```python
from build123d import *

# Parameters (mm, degrees)
RESSALTO_EXTRUS_O1_DEPTH                            = 22.5
CHANFRO1_SIZE                                       = 9
CORTE_EXTRUS_O1_REACH                               = 24.5
ESBO_O3_W                                           = 1139.230904301
ESBO_O3_H                                           = 709.798033895
CORTE_EXTRUS_O5_DEPTH                               = 1.5
CORTE_EXTRUS_O6_REACH                               = 23
ESCAREADO_PARA_PARAFUSO_ALLEN_SEXTAVADO_D           = 4.5
ESCAREADO_PARA_PARAFUSO_ALLEN_SEXTAVADO_CSINK_D     = 8.96
ESCAREADO_PARA_PARAFUSO_ALLEN_SEXTAVADO_CSINK_ANGLE = 90
CORTE_EXTRUS_O7_DEPTH                               = 10


with BuildPart() as part:
    # Esboço1 → Ressalto-extrusão1 (new body, symmetric)
    with BuildSketch(Plane.XY):
        with BuildLine():
            Line((-62.301435521, 279.499553668), (62.301435521, 279.499553668))
            ThreePointArc((62.301435521, 279.499553668), (66.527618138, 278.562631538), (69.961879952, 275.927429764))
            Line((69.961879952, 275.927429764), (100.660444431, 239.342305259))
            ThreePointArc((100.660444431, 239.342305259), (102.396926208, 236.334630596), (103, 232.914429162))
            Line((103, 232.914429162), (103, 177.526516487))
            ThreePointArc((103, 177.526516487), (102.453136861, 174.425101506), (100.878507208, 171.697762944))
            Line((100.878507208, 171.697762944), (62.121492792, 125.508951777))
            ThreePointArc((62.121492792, 125.508951777), (60.546863139, 122.781613215), (60, 119.680198234))
            Line((60, 119.680198234), (60, 5.944191717))
            Line((60, 5.944191717), (52.319579452, -0.500446332))
            Line((52.319579452, -0.500446332), (-52.319579452, -0.500446332))
            Line((-52.319579452, -0.500446332), (-60, 5.944191717))
            Line((-60, 5.944191717), (-60, 119.680198234))
            ThreePointArc((-60, 119.680198234), (-60.546863139, 122.781613215), (-62.121492792, 125.508951777))
            Line((-62.121492792, 125.508951777), (-100.878507208, 171.697762944))
            ThreePointArc((-100.878507208, 171.697762944), (-102.453136861, 174.425101506), (-103, 177.526516487))
            Line((-103, 177.526516487), (-103, 232.914429162))
            ThreePointArc((-103, 232.914429162), (-102.396926208, 236.334630596), (-100.660444431, 239.342305259))
            Line((-100.660444431, 239.342305259), (-69.961879952, 275.927429764))
            ThreePointArc((-69.961879952, 275.927429764), (-66.527618138, 278.562631538), (-62.301435521, 279.499553668))
        make_face()
        Polygon((-52.721623425, 259.499553668), (52.721623425, 259.499553668), (83, 223.415189606), (83, 181.505464287), (35, 124.301291842), (35, 19.499553668), (-35, 19.499553668), (-35, 124.301291842), (-83, 181.505464287), (-83, 223.415189606), align=None, mode=Mode.SUBTRACT)
    extrude(amount=RESSALTO_EXTRUS_O1_DEPTH, both=True)

    # Chanfro1
    chanfro1_edges = [part.edges().sort_by_distance(p)[0] for p in [
        (0, -0.500446332, 22.5),
        (56.159789726, 2.721872692, 22.5),
        (60, 62.812194975, 22.5),
        (60.546863139, 122.781613215, 22.5),
        (81.5, 148.603357361, 22.5),
        (102.453136861, 174.425101506, 22.5),
        (103, 205.220472825, 22.5),
        (102.396926208, 236.334630596, 22.5),
        (85.311162192, 257.634867512, 22.5),
        (66.527618138, 278.562631538, 22.5),
        (0, 279.499553668, 22.5),
        (-66.527618138, 278.562631538, 22.5),
        (-85.311162192, 257.634867512, 22.5),
        (-102.396926208, 236.334630596, 22.5),
        (-103, 205.220472825, 22.5),
        (-102.453136861, 174.425101506, 22.5),
        (-81.5, 148.603357361, 22.5),
        (-60.546863139, 122.781613215, 22.5),
        (-60, 62.812194975, 22.5),
        (-56.159789726, 2.721872692, 22.5),
    ]]
    chamfer(chanfro1_edges, length=CHANFRO1_SIZE)

    # Esboço3 → Corte-extrusão1 (cut, up to next)
    with BuildSketch(Plane.XY, mode=Mode.PRIVATE) as corte_extrus_o1_sk1:
        with Locations((-153.157436203, 152.53565808)):
            Rectangle(ESBO_O3_W, ESBO_O3_H)
    corte_extrus_o1_tool1 = extrude(corte_extrus_o1_sk1.sketch, amount=-CORTE_EXTRUS_O1_REACH, mode=Mode.PRIVATE) & part.part
    add(corte_extrus_o1_tool1.solids().sort_by_distance((-153.157436, 152.535658, 0))[0], mode=Mode.SUBTRACT)

    # Esboço4 → Corte-extrusão5 (cut)
    with BuildSketch(Plane.XY.offset(22.5)):
        Polygon((62.301435521, 269.499553668), (-62.301435521, 269.499553668), (-93, 232.914429162), (-93, 177.865761944), (-50, 126.620357463), (-50, 10.607268298), (-48.679877109, 9.499553668), (48.679877109, 9.499553668), (50, 10.607268298), (50, 126.620357463), (93, 177.865761944), (93, 232.914429162), align=None)
        Polygon((35, 19.499553668), (-35, 19.499553668), (-35, 124.301291842), (-83, 181.505464287), (-83, 223.415189606), (-52.721623425, 259.499553668), (52.721623425, 259.499553668), (83, 223.415189606), (83, 181.505464287), (35, 124.301291842), align=None, mode=Mode.SUBTRACT)
    extrude(amount=-CORTE_EXTRUS_O5_DEPTH, mode=Mode.SUBTRACT)

    # Esboço5 → Corte-extrusão6 (cut, up to next)
    with BuildSketch(Plane.XY.offset(21), mode=Mode.PRIVATE) as corte_extrus_o6_sk1:
        Polygon((-93, 232.914429162), (-83, 223.415189606), (-83, 181.505464287), (-35, 124.301291842), (-35, 108.744053574), (-93, 177.865761944), align=None)
    corte_extrus_o6_tool1 = extrude(corte_extrus_o6_sk1.sketch, amount=-CORTE_EXTRUS_O6_REACH, mode=Mode.PRIVATE) & part.part
    add(corte_extrus_o6_tool1.solids().sort_by_distance((-88.943881, 227.171171, 21))[0], mode=Mode.SUBTRACT)
    # Esboço5 → Corte-extrusão6 (cut, up to next)
    with BuildSketch(Plane.XY.offset(21), mode=Mode.PRIVATE) as corte_extrus_o6_sk2:
        Polygon((-52.721623425, 259.499553668), (-62.301435521, 269.499553668), (62.301435521, 269.499553668), (52.721623425, 259.499553668), align=None)
    corte_extrus_o6_tool2 = extrude(corte_extrus_o6_sk2.sketch, amount=-CORTE_EXTRUS_O6_REACH, mode=Mode.PRIVATE) & part.part
    add(corte_extrus_o6_tool2.solids().sort_by_distance((0, 264.638364, 21))[0], mode=Mode.SUBTRACT)
    # Esboço5 → Corte-extrusão6 (cut, up to next)
    with BuildSketch(Plane.XY.offset(21), mode=Mode.PRIVATE) as corte_extrus_o6_sk3:
        Polygon((-50, 10.607268298), (-35, 19.499553668), (35, 19.499553668), (50, 10.607268298), (48.679877109, 9.499553668), (-48.679877109, 9.499553668), align=None)
    corte_extrus_o6_tool3 = extrude(corte_extrus_o6_sk3.sketch, amount=-CORTE_EXTRUS_O6_REACH, mode=Mode.PRIVATE) & part.part
    add(corte_extrus_o6_tool3.solids().sort_by_distance((0, 14.193497, 21))[0], mode=Mode.SUBTRACT)
    # Esboço5 → Corte-extrusão6 (cut, up to next)
    with BuildSketch(Plane.XY.offset(21), mode=Mode.PRIVATE) as corte_extrus_o6_sk4:
        Polygon((35, 108.744053574), (93, 177.865761944), (93, 232.914429162), (83, 223.415189606), (83, 181.505464287), (35, 124.301291842), align=None)
    corte_extrus_o6_tool4 = extrude(corte_extrus_o6_sk4.sketch, amount=-CORTE_EXTRUS_O6_REACH, mode=Mode.PRIVATE) & part.part
    add(corte_extrus_o6_tool4.solids().sort_by_distance((62.950148, 144.185838, 21))[0], mode=Mode.SUBTRACT)

    # Escareado para parafuso Allen sextavado escareado de M41 (through all)
    with Locations(Plane(origin=(-66.589178595, 253.499553668, 22.5), x_dir=(1, 0, 0), z_dir=(0, 0, 1))):
        with Locations((0, 0), (-10.908295205, -13), (133.17835719, 0), (144.086652395, -13), (24.089178595, -199), (24.089178595, -229), (109.089178595, -229), (109.089178595, -199)):
            CounterSinkHole(ESCAREADO_PARA_PARAFUSO_ALLEN_SEXTAVADO_D / 2, ESCAREADO_PARA_PARAFUSO_ALLEN_SEXTAVADO_CSINK_D / 2, counter_sink_angle=ESCAREADO_PARA_PARAFUSO_ALLEN_SEXTAVADO_CSINK_ANGLE)

    # Esboço9 → Corte-extrusão7 (cut)
    with BuildSketch(Plane(origin=(0, 0, 0), x_dir=(-1, 0, 0), z_dir=(0, 0, -1))):
        Polygon((-66.589178595, 257.541005552), (-70.089178595, 255.52027961), (-70.089178595, 251.478827725), (-66.589178595, 249.458101783), (-63.089178595, 251.478827725), (-63.089178595, 255.52027961), align=None)
        Polygon((-77.4974738, 244.541005552), (-80.9974738, 242.52027961), (-80.9974738, 238.478827725), (-77.4974738, 236.458101783), (-73.9974738, 238.478827725), (-73.9974738, 242.52027961), align=None)
        Polygon((-42.5, 58.541005552), (-46, 56.52027961), (-46, 52.478827725), (-42.5, 50.458101783), (-39, 52.478827725), (-39, 56.52027961), align=None)
        Polygon((-42.5, 28.541005552), (-46, 26.52027961), (-46, 22.478827725), (-42.5, 20.458101783), (-39, 22.478827725), (-39, 26.52027961), align=None)
        Polygon((39, 26.52027961), (42.5, 28.541005552), (46, 26.52027961), (46, 22.478827725), (42.5, 20.458101783), (39, 22.478827725), align=None)
        Polygon((39, 56.52027961), (42.5, 58.541005552), (46, 56.52027961), (46, 52.478827725), (42.5, 50.458101783), (39, 52.478827725), align=None)
        Polygon((73.9974738, 242.52027961), (77.4974738, 244.541005552), (80.9974738, 242.52027961), (80.9974738, 238.478827725), (77.4974738, 236.458101783), (73.9974738, 238.478827725), align=None)
        Polygon((63.089178595, 255.52027961), (66.589178595, 257.541005552), (70.089178595, 255.52027961), (70.089178595, 251.478827725), (66.589178595, 249.458101783), (63.089178595, 251.478827725), align=None)
    extrude(amount=-CORTE_EXTRUS_O7_DEPTH, mode=Mode.SUBTRACT)


solid = part.part
```
Here's how the part is built. I have some questions about the finished solid (model axes, mm). A direction names the side the tool comes from. Round coordinates to 2 decimals unless told otherwise and drop trailing zeros. Order: outer loops, then holes, each group sorted by start corner. A loop starts at its lowest first (then second) coordinate and runs counter-clockwise, first axis right, second up. Notation, with made-up numbers: M 62.5,9 L 66.5,9 A26 cw 66.5,30 Z; hole C 77.5,88.25 d1. An arc over 180 degrees is marked long. Answer in a Markdown table with one row per item.
Item 1: Imagine slicing it at B-B, the plane z = 4.5. State how many separate pieces and enclosed holes the cut face has, and give its area (3 significant figures).
A:
| item | result |
|---|---|
| separate pieces | 1 |
| enclosed holes | 9 |
| area | 12,300 mm2 |
Item 2: For faces 1 (the face through (75, 241, 10)), 2 (the face through (-82.127, 254.527, 17.937)), 3 (the face through (-77.44, 251.46, 21.76)), which set-ups out of +Z, -Z, +X, -X, +Y, -Y let a thin tool reach every point of the face, with its end or its side?
A:
| item | result |
|---|---|
| face 1 | -Z |
| face 2 | +Z, -X, +Y |
| face 3 | +Z |
Item 3: If I drill on L1, parallel to Y at x = -42.5, z = 17.75; L2, parallel to Y at x = -42.5, z = 17.25; L3, parallel to X at y = 189, z = 4.5, over which ranges is the centre line in solid material (lowest first)? Write a range as from..to.
A:
| item | result |
|---|---|
| L1 | y = 3.75..9.5, 15.05..22.25, 26.75..52.25, 56.75..117.68, 269.5..275.25 |
| L2 | y = 3.25..9.5, 15.05..22.25, 26.75..52.25, 56.75..117.68, 269.5..275.75 |
| L3 | x = -103..-93, 93..103 |
Item 4: Imagine slicing it at A-A, the plane y = 153.5. Write out the boundary of the cut face in (x, z).
A:
| item | result |
|---|---|
| outline | M -85.61,0 L -72.55,0 L -72.55,22.5 L -73.86,22.5 L -85.61,13.5 Z; M 72.55,0 L 85.61,0 L 85.61,13.5 L 73.86,22.5 L 72.55,22.5 Z |
Item 5: I'm going to push flat-ended pins straight in: pin 1 (3 mm diameter, centred on y = 253.5, z = 5, fed in from -X); pin 2 (10.5 mm diameter, centred on y = 71, z = 6.5, fed in from -X); pin 3 (6 mm diameter, centred on x = -81.5, z = 7.5, fed in from -Y); pin 4 (7.5 mm diameter, centred on x = -67, y = 254, fed in from -Z). Where does each tip first touch, or does it pass through?
A:
| item | result |
|---|---|
| pin 1 | stops at x = -90.04 |
| pin 2 | stops at x = -60 |
| pin 3 | stops at y = 145.03 |
| pin 4 | stops at z = 0 |
Item 6: Thinking about a two-plate mould opening in X: for faces 4 (the face through (73, 247, 21)), 5 (the face through (-1, 275, 18)), 6 (the face through (85.096, 257.891, 6.844)), 7 (the face through (-35, 63, 11)), which applies, +X half, -X half, draft (parallel to the pull), parting line (faces both ways), or undercut?
A:
| item | result |
|---|---|
| face 4 | undercut |
| face 5 | draft |
| face 6 | +X half |
| face 7 | undercut |
